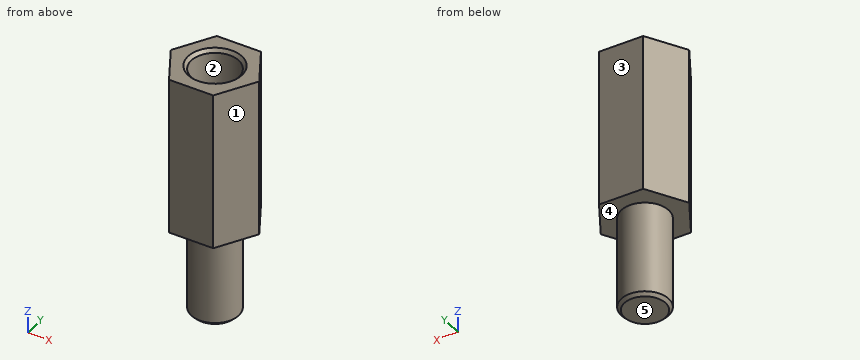
```python
from build123d import *

# Parameters (mm, degrees)
PAD_DEPTH    = 10
SKETCH001_R  = 1.5
PAD001_DEPTH = 6
SKETCH002_R  = 1.5
POCKET_DEPTH = 6
CHAMFER_SIZE = 0.2


with BuildPart() as part:
    # Sketch → Pad (new body)
    with BuildSketch(Plane.XY):
        Polygon((2.8, 0), (1.4, 2.424871), (-1.4, 2.424871), (-2.8, 0), (-1.4, -2.424871), (1.4, -2.424871), align=None)
    extrude(amount=PAD_DEPTH)

    # Sketch001 (on Face7 of Pad) → Pad001 (join)
    with BuildSketch(Plane(origin=(0, 0, 0), x_dir=(1, 0, 0), z_dir=(0, 0, -1))):
        Circle(SKETCH001_R)
    extrude(amount=PAD001_DEPTH)

    # Sketch002 (on Face5 of Pad001) → Pocket (cut)
    with BuildSketch(Plane.XY.offset(10)):
        Circle(SKETCH002_R)
    extrude(amount=-POCKET_DEPTH, mode=Mode.SUBTRACT)

    # Chamfer
    chamfer_edges = [part.edges().sort_by_distance(p)[0] for p in [
        (-1.5, 0, 10),
        (-1.5, 0, -6),
    ]]
    chamfer(chamfer_edges, length=CHAMFER_SIZE)


solid = part.part
```
Model file for the job. Use its own axes, mm. Face numbers are marked on the shaded views. A direction names the side the tool comes from. Give positions to 0.01 mm unless a question says otherwise; leave off trailing zeros. Write each loop counter-clockwise with the first axis right and the second up, starting at its lowest first coordinate (ties: lowest second). Pieces come first, ordered by that corner, then holes. Notation, with made-up numbers: (64, 88.5) -> (83, 88.5) arc R17 cw to (83, 119.5) -> close; hole circle Ø1 at (-32.75, -2.75). An arc over 180 degrees is marked (long way). Use CSV: the item, a comma, the result in double quotes. Start each with the question number.
1) Drill centre lines: L1, parallel to Y at x = 0, z = 6.15; L2, parallel to Z at x = 0.1, y = 1.25; L3, parallel to Z at x = 1.75, y = -1.45. Where is each one in solid material? Low to high.
2) Cut at A-A on x = 0. List the corners of the cut face in (y, z), plus the area to 3 significant figures.
3) Cut at C-C on z = -1. List the corners of the cut face in (x, y).
4) Pin check, flat tips, straight feed: P1, Ø1.5, axis at x = 0.5, y = -0.5, coming from the +Z side; P2, Ø1.5, axis at x = -2, y = 1.5, coming from the -Z side; P3, Ø1.5, axis at y = 1, z = 7, coming from the -X side. Stop position of each tip, or through.
5) Cut at D-D on x = -2.4. List the corners of the cut face in (y, z), plus the area to 3 significant figures.
6) Two-plate mould, pull along X, no slides. Class the marked faces 1, 2 and 3: released by +X, released by -X, zero draft, split by the parting line, or undercut.
7) Tool access for the marked faces 4 and 5: list every direction of +Z, -Z, +X, -X, +Y, -Y with a clear straight run to the whole face (end or side of a thin tool).
8) Cut at B-B on z = 2.5. List the corners of the cut face in (x, y), plus the area to 3 significant figures.
Final values:
1,L1,"y = -2.42 to -1.5, 1.5 to 2.42"
1,L2,"z = -6 to 4"
1,L3,"z = 0 to 10"
2,outline,"(-2.42, 0) -> (-1.5, 0) -> (-1.5, -5.8) -> (-1.3, -6) -> (1.3, -6) -> (1.5, -5.8) -> (1.5, 0) -> (2.42, 0) -> (2.42, 10) -> (1.7, 10) -> (1.5, 9.8) -> (1.5, 4) -> (-1.5, 4) -> (-1.5, 9.8) -> (-1.7, 10) -> (-2.42, 10) -> close"
2,area,"48.4 mm2"
3,outline,"circle Ø3 at (0, 0)"
4,P1,"stops at z = 4"
4,P2,"stops at z = 0"
4,P3,"stops at x = -2.66"
5,outline,"(-0.69, 0) -> (0.69, 0) -> (0.69, 10) -> (-0.69, 10) -> close"
5,area,"13.9 mm2"
6,face 1,"released by +X"
6,face 2,"undercut"
6,face 3,"zero draft"
7,face 4,"-Z"
7,face 5,"-Z, +X, -X, +Y, -Y"
8,outline,"(-2.8, 0) -> (-1.4, -2.42) -> (1.4, -2.42) -> (2.8, 0) -> (1.4, 2.42) -> (-1.4, 2.42) -> close"
8,area,"20.4 mm2"
